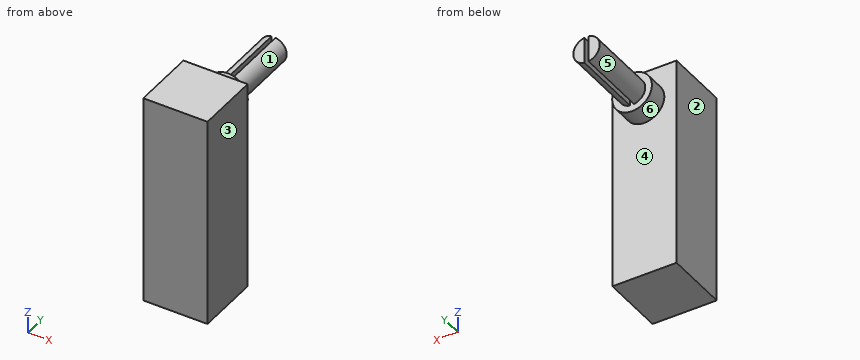
```python
from build123d import *

# Parameters (mm, degrees)
SKETCH1_W           = 12.319
SKETCH1_H           = 12.319
BOSS_EXTRUDE1_DEPTH = 40.64
BOSS_EXTRUDE2_DEPTH = 17.78
SKETCH3_R           = 3.81
BOSS_EXTRUDE3_DEPTH = 3.81


with BuildPart() as part:
    # Sketch1 → Boss-Extrude1 (new body)
    with BuildSketch(Plane.XY):
        with Locations((0, -6.1595)):
            Rectangle(SKETCH1_W, SKETCH1_H)
    extrude(amount=BOSS_EXTRUDE1_DEPTH)

    # Sketch2 → Boss-Extrude2 (add)
    with BuildSketch(Plane(origin=(0, 0, 0), x_dir=(1, 0, 0), z_dir=(0, 1, 0))):
        with BuildLine():
            Line((-0.381, -31.778737568), (-0.381, -36.801262432))
            ThreePointArc((-0.381, -36.801262432), (-2.54, -34.29), (-0.381, -31.778737568))
        make_face()
        with BuildLine():
            Line((0.381, -31.778737568), (0.381, -36.801262432))
            ThreePointArc((0.381, -36.801262432), (2.54, -34.29), (0.381, -31.778737568))
        make_face()
    extrude(amount=BOSS_EXTRUDE2_DEPTH)

    # Sketch3 → Boss-Extrude3 (add)
    with BuildSketch(Plane(origin=(0, 0, 0), x_dir=(1, 0, 0), z_dir=(0, 1, 0))):
        with Locations((0, -34.29)):
            Circle(SKETCH3_R)
    extrude(amount=BOSS_EXTRUDE3_DEPTH)


solid = part.part
```
Design review of the part built by this model. Coordinates are the model's own, in mm. Face numbers are marked on the shaded views. A direction names the side the tool comes from. Give positions to 0.01 mm unless a question says otherwise; leave off trailing zeros. Order: outer loops, then holes, each group sorted by start corner. A loop starts at its lowest first (then second) coordinate and runs counter-clockwise, first axis right, second up. Notation, with made-up numbers: M 3.25,41 L 27.25,41 A13 ccw 27.25,58 Z; hole C 86,-4 d5. An arc over 180 degrees is marked long. One line per question, with ' | ' between items. Start each with the question number.
Q1. We need section C-C (x = -3.25). Write out the cut boundary in (y, z).
Q2. For pin 1 Ø5.5 at (y, z) = (12.5, 34.5) entering from +X; pin 2 Ø4 at (y, z) = (14, 33) entering from -X; pin 3 Ø2 at (x, z) = (2, 11.5) entering from +Y, all flat-tipped, find the tip position at first contact; note any pin that passes through.
Q3. We need section D-D (y = 0.5). Write out the cut boundary in (x, z), plus the area to 3 significant figures.
Q4. For L1, parallel to Y at x = -3.5, z = 2.5; L2, parallel to X at y = 15.5, z = 33; L3, parallel to Y at x = -2.25, z = 37, list the stretches that pass through material, from the lowest coordinate up. Write a range as [from, to].
Q5. Machinability: for the marked faces 1 and 2, which of the approach directions +Z, -Z, +X, -X, +Y, -Y give a long, thin tool a straight path to every point of the face, cutting with its end or side? Answer none if there is none.
Q6. The part is to be moulded in two halves that separate along X. For the marked faces 3, 4, 5 and 6, say which applies: +X half, -X half, draft (parallel to the pull), parting line (faces both ways), or undercut.
Q7. We need section A-A (z = 34.29). Write out the cut boundary in (x, y), plus the area to 3 significant figures.
Q8. We need section B-B (y = 12). Write out the cut boundary in (x, z).
Returned:
1) outline: M -12.32,0 L 0,0 L 0,32.3 L 3.81,32.3 L 3.81,36.28 L 0,36.28 L 0,40.64 L -12.32,40.64 Z
2) pin 1: x = 2.54 | pin 2: x = -2.54 | pin 3: y = 0
3) outline: C 0,34.29 d7.62 | area: 45.6 mm2
4) L1: [-12.32, 0] | L2: [-2.19, -0.38], [0.38, 2.19] | L3: [-12.32, 3.81]
5) face 1: +X, +Y | face 2: +Z, -Z, -X, +Y, -Y
6) face 3: +X half | face 4: draft | face 5: -X half | face 6: parting line
7) outline: M -6.16,-12.32 L 6.16,-12.32 L 6.16,0 L 3.81,0 L 3.81,3.81 L 2.54,3.81 L 2.54,17.78 L 0.38,17.78 L 0.38,3.81 L -0.38,3.81 L -0.38,17.78 L -2.54,17.78 L -2.54,3.81 L -3.81,3.81 L -3.81,0 L -6.16,0 Z | area: 241 mm2
8) outline: M -0.38,31.78 L -0.38,36.8 A2.54 ccw Z; M 0.38,31.78 A2.54 ccw 0.38,36.8 Z
